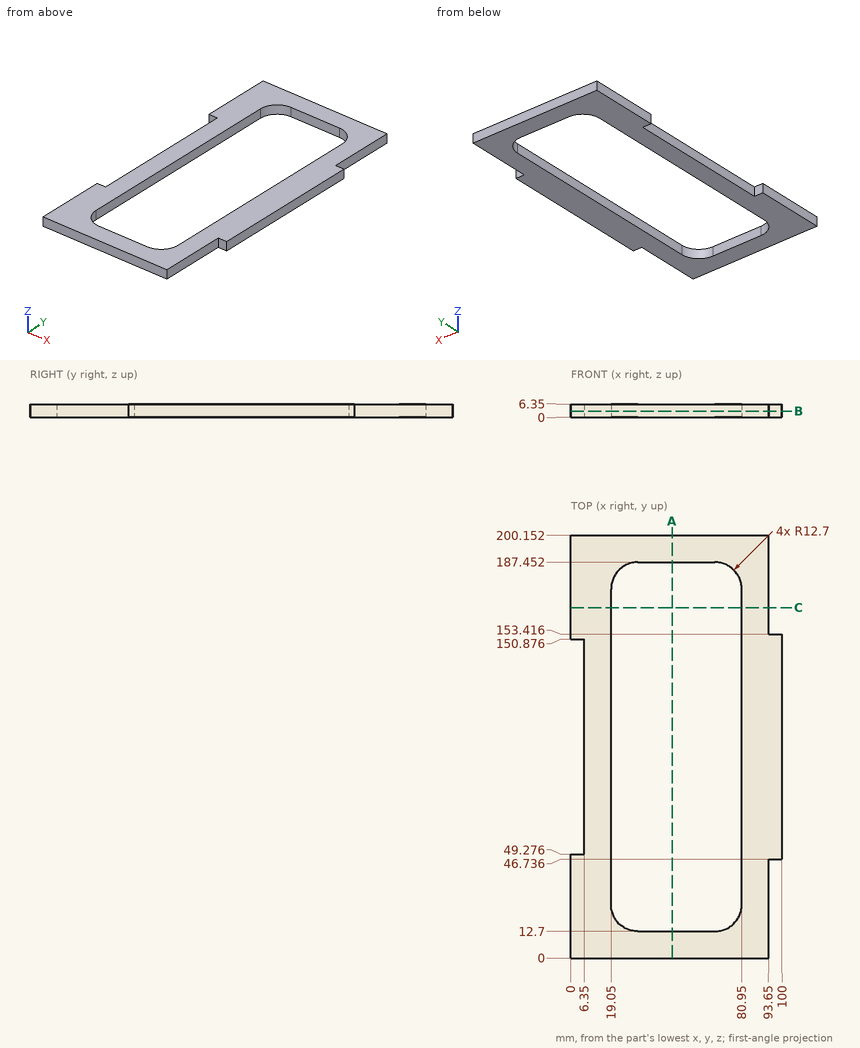
The figure shows three views and two pictorial views of one solid part (mm, origin at its lowest corner). Answer the questions. Give positions to 0.01 mm unless a question says otherwise; leave off trailing zeros. Write each loop counter-clockwise with the first axis right and the second up, starting at its lowest first coordinate (ties: lowest second). Pieces come first, ordered by that corner, then holes. Notation, with made-up numbers: M -7.75,80.25 L 2.25,80.25 A7 ccw 2.25,90.25 Z; hole C 33,19 d11. An arc over 180 degrees is marked long. Write each question's results on one line, items separated by ' | '.
Q1. Flat-ended cylindrical pins translate along their axes: P1, Ø1, axis at y = 109.5, z = 5, coming from the -X side; P2, Ø3, axis at y = 29.5, z = 2.5, coming from the +X side; P3, Ø3, axis at x = 97.5, z = 2, coming from the +Y side. Find the tip coordinate at first contact, or state that the pin passes through.
Output values:
P1: x = 6.35 | P2: x = 93.65 | P3: y = 153.42
Q2. Section A-A, the plane x = 48 is taken. Write down the section's boundary in (y, z).
Output values:
outline: M 0,0 L 12.7,0 L 12.7,6.35 L 0,6.35 Z; M 187.45,0 L 200.15,0 L 200.15,6.35 L 187.45,6.35 Z
Q3. Section B-B, the plane z = 3 is taken. Write down the section's boundary in (x, y), then the cut area to 3 significant figures.
Output values:
outline: M 0,0 L 93.65,0 L 93.65,46.74 L 100,46.74 L 100,153.42 L 93.65,153.42 L 93.65,200.15 L 0,200.15 L 0,150.88 L 6.35,150.88 L 6.35,49.28 L 0,49.28 Z; hole M 19.05,25.4 A12.7 ccw 31.75,12.7 L 68.25,12.7 A12.7 ccw 80.95,25.4 L 80.95,174.75 A12.7 ccw 68.25,187.45 L 31.75,187.45 A12.7 ccw 19.05,174.75 Z | area: 8,100 mm2
Q4. Section C-C, the plane y = 166 is taken. Write down the section's boundary in (x, z), then the cut area to 3 significant figures.
Output values:
outline: M 0,0 L 19.05,0 L 19.05,6.35 L 0,6.35 Z; M 80.95,0 L 93.65,0 L 93.65,6.35 L 80.95,6.35 Z | area: 202 mm2
Q5. Consider L1, parallel to X at y = 75, z = 1; L2, parallel to Y at x = 53, z = 5.25; L3, parallel to X at y = 173.5, z = 3.5. Determine where each line is inside the solid, lowest interval first. Write a range as from..to.
Output values:
L1: 6.35..19.05, 80.95..100 | L2: 0..12.7, 187.45..200.15 | L3: 0..19.05, 80.95..93.65
